```python
from build123d import *

# Parameters (mm, degrees)
BOSS_EXTRUDE1_DEPTH      = 37.5
BOSS_EXTRUDE1_DEPTH_BACK = 37.5
SKETCH2_R                = 50
BOSS_EXTRUDE2_DEPTH      = 112.5
BOSS_EXTRUDE2_DEPTH_BACK = 112.5
BOSS_EXTRUDE3_DEPTH      = 12.5
BOSS_EXTRUDE3_DEPTH_BACK = 12.5
BOSS_EXTRUDE4_DEPTH      = 12.5
BOSS_EXTRUDE4_DEPTH_BACK = 12.5


with BuildPart() as part:
    # Sketch2 → Boss-Extrude1 (new, two sides: drawn at the far end of the back side and taken through both)
    with BuildSketch(Plane(origin=(0, 0, 0), x_dir=(0, 0, -1), z_dir=(1, 0, 0)).offset(-BOSS_EXTRUDE1_DEPTH_BACK)):
        with BuildLine():
            Line((0, 150), (150, 150))
            Line((150, 150), (150, -150))
            Line((150, -150), (0, -150))
            ThreePointArc((0, -150), (-150, 0), (0, 150))
        make_face()
        Circle(SKETCH2_R, mode=Mode.SUBTRACT)
    extrude(amount=BOSS_EXTRUDE1_DEPTH + BOSS_EXTRUDE1_DEPTH_BACK)

    # Sketch2_12 → Boss-Extrude2 (add, two sides: drawn at the far end of the back side and taken through both)
    with BuildSketch(Plane(origin=(0, 0, 0), x_dir=(0, 0, -1), z_dir=(1, 0, 0)).offset(-BOSS_EXTRUDE2_DEPTH_BACK)):
        Polygon((375, -150), (150, -150), (150, 150), (375, 150), (375, 100), (250, 100), (250, -100), (375, -100), align=None)
    extrude(amount=BOSS_EXTRUDE2_DEPTH + BOSS_EXTRUDE2_DEPTH_BACK)

    # Sketch2_13 → Boss-Extrude3 (add, two sides: drawn at the far end of the back side and taken through both)
    with BuildSketch(Plane(origin=(0, 0, 0), x_dir=(0, 0, -1), z_dir=(1, 0, 0)).offset(-BOSS_EXTRUDE3_DEPTH_BACK)):
        Polygon((375, 100), (375, 75), (450, 75), (450, 150), (375, 150), align=None)
    extrude(amount=BOSS_EXTRUDE3_DEPTH + BOSS_EXTRUDE3_DEPTH_BACK)

    # Sketch2_14 → Boss-Extrude4 (add, two sides: drawn at the far end of the back side and taken through both)
    with BuildSketch(Plane(origin=(0, 0, 0), x_dir=(0, 0, -1), z_dir=(1, 0, 0)).offset(-BOSS_EXTRUDE4_DEPTH_BACK)):
        Polygon((450, -150), (375, -150), (375, -100), (375, -25), (450, -25), align=None)
    extrude(amount=BOSS_EXTRUDE4_DEPTH + BOSS_EXTRUDE4_DEPTH_BACK)


solid = part.part
```
Check sheet for the modelled part. Datum: model origin and axes. Units: mm. A direction names the side the tool comes from. Round coordinates to 2 decimals unless told otherwise and drop trailing zeros. Order: outer loops, then holes, each group sorted by start corner. A loop starts at its lowest first (then second) coordinate and runs counter-clockwise, first axis right, second up.
1) Scan lines: line 1 (Y direction, x = 65, z = -293); line 2 (X direction, y = -83, z = -120); line 3 (Z direction, x = 92.5, y = -79). Record each from-to range of solid material in increasing order.
2) Section check B-B (z = -256). Record the boundary of the cut face in (x, y).
3) Section check A-A (y = 0). Record the boundary of the cut face in (x, z), and give its area (3 significant figures).
4) Section check C-C (x = -27.5). Record the boundary of the cut face in (y, z).
5) Section check D-D (x = 55). Record the boundary of the cut face in (y, z), and give its area (3 significant figures).
6) Mould release check, pull along Z, two halves, no side actions. Record for faces 1 (the flat face through (62, -125, -375)), 2 (the flat face through (0, -62, -375)), 3 (the flat face through (-76, -2, -150)): +Z half, -Z half, draft (parallel to the pull), parting line (faces both ways), or undercut.
7) Go/stop test with flat-tipped pins: pin 1 Ø12.5 at (x, y) = (5.5, -60) entering from +Z; pin 2 Ø12 at (x, y) = (-86, 36) entering from +Z; pin 3 Ø4 at (y, z) = (80, -375) entering from +X. Record where each tip stops, or that it passes through.
8) Tool access check on faces 4 (the flat face through (0, -25, -412)), 5 (the flat face through (-63, 125, -375)), 6 (the flat face through (12.5, 113, -412)). Record the directions out of +Z, -Z, +X, -X, +Y, -Y that give a thin tool (end or side, any length) a straight path to the whole face; none if there is none.
Result:
1. line 1: y = -150 to -100, 100 to 150
1. line 2: x = -37.5 to 37.5
1. line 3: z = -250 to -150
2. outline: (-112.5, -150) - (112.5, -150) - (112.5, -100) - (-112.5, -100) - close; (-112.5, 100) - (112.5, 100) - (112.5, 150) - (-112.5, 150) - close
3. outline: (-112.5, -250) - (112.5, -250) - (112.5, -150) - (37.5, -150) - (37.5, -50) - (-37.5, -50) - (-37.5, -150) - (-112.5, -150) - close; (-37.5, 50) - (37.5, 50) - (37.5, 150) - (-37.5, 150) - close
3. area: 37,500 mm2
4. outline: (-150, -375) - (-100, -375) - (-100, -250) - (100, -250) - (100, -375) - (150, -375) - (150, 0) arc R150 ccw to (-150, 0) - close; hole circle Ø100 at (0, 0)
5. outline: (-150, -375) - (-100, -375) - (-100, -250) - (100, -250) - (100, -375) - (150, -375) - (150, -150) - (-150, -150) - close
5. area: 42,500 mm2
6. face 1: -Z half
6. face 2: undercut
6. face 3: +Z half
7. pin 1: stops at z = 140.04
7. pin 2: stops at z = -150
7. pin 3: stops at x = 12.5
8. face 4: -Z, +X, -X
8. face 5: -Z, -X, +Y, -Y
8. face 6: -Z, +X, +Y, -Y
